```python
from build123d import *

# Parameters (mm, degrees)
F1_DEPTH = 35
F2_R     = 2


with BuildPart() as f1:
    # F0 (on Top) → F1 (new body)
    with BuildSketch(Plane.XY):
        with BuildLine():
            Line((0, 50), (0, 0))
            Line((0, 0), (3, 0))
            Line((3, 0), (3, 46))
            Line((3, 46), (23, 46))
            Line((23, 46), (23, -60))
            ThreePointArc((23, -60), (36, -73), (49, -60))
            Line((49, -60), (46, -60))
            ThreePointArc((46, -60), (36, -70), (26, -60))
            Line((26, -60), (26, 50))
            Line((26, 50), (0, 50))
        make_face()
    extrude(amount=F1_DEPTH)

    # F2
    f2_edges = [f1.edges().sort_by_distance(p)[0] for p in [
        (47.5, -60, 35),
        (47.5, -60, 0),
        (1.5, 0, 35),
        (1.5, 0, 0),
    ]]
    fillet(f2_edges, radius=F2_R)


solid = f1.part
```
For this review, take the finished solid that the model builds, in its own axes (mm). A direction names the side the tool comes from. Coordinates: 2 decimals unless noted, no trailing zeros. Write each loop counter-clockwise with the first axis right and the second up, starting at its lowest first coordinate (ties: lowest second). Pieces come first, ordered by that corner, then holes. Notation, with made-up numbers: (49.25, 82) - (68.25, 82) arc R33 cw to (68.25, 110) - close; hole circle Ø9 at (30.5, -34.5). An arc over 180 degrees is marked (long way). Put each result on its own line as item: value.
1. Wall thickness on probe 1 along X at (y, z) = (32, 26.5); probe 2 along Y at (x, z) = (10, 16); probe 3 along X at (y, z) = (-47.5, 4.5): over which ranges is each line inside the solid? List them lowest first.
Values found:
probe 1: 0 to 3, 23 to 26
probe 2: 46 to 50
probe 3: 23 to 26
2. Add section B-B, the plane z = 7.5. Give the boundary of the cut face in (x, y).
Values found:
outline: (0, 0) - (3, 0) - (3, 46) - (23, 46) - (23, -60) arc R13 ccw to (49, -60) - (46, -60) arc R10 cw to (26, -60) - (26, 50) - (0, 50) - close
3. Add section C-C, the plane x = 36. Give the boundary of the cut face in (y, z).
Values found:
outline: (-73, 0) - (-70, 0) - (-70, 35) - (-73, 35) - close
4. Add section D-D, the plane y = -54. Give the boundary of the cut face in (x, z), then the cut area to 3 significant figures.
Values found:
outline: (23, 0) - (26, 0) - (26, 35) - (23, 35) - close
area: 105 mm²
5. Machinability: for faces 4 (the flat face through (26, -6, 17)), 5 (the flat face through (1, 0, 17)), 6 (the flat face through (13, 46, 17)), which of the approach directions +Z, -Z, +X, -X, +Y, -Y give a long, thin tool a straight path to every point of the face, cutting with its end or side? Answer none if there is none.
Values found:
face 4: +Z, -Z, +X, +Y
face 5: +Z, -Z, -X, -Y
face 6: +Z, -Z, -Y
6. Mouldability with a two-part tool opening along X and no side actions: class faces 1 (the cylindrical face through (36, -73, 17)), 2 (the flat face through (13, 50, 17)), 3 (the flat face through (23, -6, 17)) as released by +X, released by -X, zero draft, split by the parting line, or undercut.
Values found:
face 1: split by the parting line
face 2: zero draft
face 3: undercut
7. Add section A-A, the plane y = 40.5. Give the boundary of the cut face in (x, z).
Values found:
outline: (0, 0) - (3, 0) - (3, 35) - (0, 35) - close; (23, 0) - (26, 0) - (26, 35) - (23, 35) - close
8. For pin 1 (16 mm diameter, centred on x = 14, z = 24, fed in from -Y); pin 2 (2.5 mm diameter, centred on x = 47, z = 12.5, fed in from +Y); pin 3 (2 mm diameter, centred on y = 8, z = 8, fed in from -X); pin 4 (1 mm diameter, centred on y = -12, z = 28.5, fed in from +X), all flat-tipped, find the tip position at first contact; note any pin that passes through.
Values found:
pin 1: y = 46
pin 2: y = -60
pin 3: x = 0
pin 4: x = 26
